For this review, take the finished solid that the model builds, in its own axes (mm). A direction names the side the tool comes from. Give positions to 0.01 mm unless a question says otherwise; leave off trailing zeros. Write each loop counter-clockwise with the first axis right and the second up, starting at its lowest first coordinate (ties: lowest second). Pieces come first, ordered by that corner, then holes.
1) We need section B-B on z = -22. Give the boundary of the cut face in (x, y), and give its area (3 significant figures).
2) We need section A-A on y = 0.7. Give the boundary of the cut face in (x, z), and give its area (3 significant figures).
3) Wall thickness on line 1 along Z through (x, y) = (4, 0.5); line 2 along X through (y, z) = (0.5, -3); line 3 along Z through (x, y) = (5.25, 0.7): over which ranges is each line inside the solid? List them lowest first.
4) For P1, Ø0.5, axis at x = 18, y = 0.5, coming from the +Z side; P2, Ø0.5, axis at y = 0.5, z = -1.5, coming from the +X side, all flat-tipped, find the tip position at first contact; note any pin that passes through.
5) Draft analysis for pull direction X (two halves, no side actions). For faces 3 (the face through (18.5, 0.5, -20.3)), 4 (the face through (2.25, 0.49, -3.08)), 5 (the face through (17.9, 0.5, -2.2)), state which applies: pulls with the +X half, pulls with the -X half, needs draft (parallel to the pull), parting line crosses it, or undercut.
6) We need section C-C on x = 4. Give the boundary of the cut face in (y, z), and give its area (3 significant figures).
7) Machinability: for faces 1 (the face through (17.3, 0.5, -1.1)), 2 (the face through (0.285, 0.507, -39.699)), which of the approach directions +Z, -Z, +X, -X, +Y, -Y give a long, thin tool a straight path to every point of the face, cutting with its end or side? Answer none if there is none.
from build123d import *

# Parameters (mm, degrees)
CROQUIS1_W              = 18.5
CROQUIS1_H              = 40
CROQUIS1_R              = 1.75
SALIENTE_EXTRUIR1_DEPTH = 1
CROQUIS2_W              = 1.2
CROQUIS2_H              = 2.2
CORTAR_EXTRUIR1_DEPTH   = 1
REDONDEO1_R             = 1


with BuildPart() as part:
    # Croquis1 → Saliente-Extruir1 (new body)
    with BuildSketch(Plane(origin=(0, 0, 0), x_dir=(1, 0, 0), z_dir=(0, 1, 0))):
        with Locations((9.25, 20)):
            Rectangle(CROQUIS1_W, CROQUIS1_H)
        with Locations((4, 3)):
            Circle(CROQUIS1_R, mode=Mode.SUBTRACT)
        with Locations((4, 22)):
            Circle(CROQUIS1_R, mode=Mode.SUBTRACT)
    extrude(amount=SALIENTE_EXTRUIR1_DEPTH)

    # Croquis2 → Cortar-Extruir1 (cut)
    with BuildSketch(Plane(origin=(0, 1, 0), x_dir=(1, 0, 0), z_dir=(0, 1, 0))):
        with Locations((17.9, 1.1)):
            Rectangle(CROQUIS2_W, CROQUIS2_H)
    extrude(amount=-CORTAR_EXTRUIR1_DEPTH, mode=Mode.SUBTRACT)

    # Redondeo1
    redondeo1_edges = [part.edges().sort_by_distance(p)[0] for p in [
        (0, 0.5, -40),
        (18.5, 0.5, -40),
    ]]
    fillet(redondeo1_edges, radius=REDONDEO1_R)


solid = part.part
Results list:
1. outline: (0, 0) - (2.25, 0) - (2.25, 1) - (0, 1) - close; (5.75, 0) - (18.5, 0) - (18.5, 1) - (5.75, 1) - close
1. area: 15.0 mm2
2. outline: (0, -39) arc R1 ccw to (1, -40) - (17.5, -40) arc R1 ccw to (18.5, -39) - (18.5, -2.2) - (17.3, -2.2) - (17.3, 0) - (0, 0) - close; hole circle Ø3.5 at (4, -22); hole circle Ø3.5 at (4, -3)
2. area: 718 mm2
3. line 1: z = -40 to -23.75, -20.25 to -4.75, -1.25 to 0
3. line 2: x = 0 to 2.25, 5.75 to 18.5
3. line 3: z = -40 to -23.22, -20.78 to -4.22, -1.78 to 0
4. P1: stops at z = -2.2
4. P2: stops at x = 17.3
5. face 3: pulls with the +X half
5. face 4: undercut
5. face 5: needs draft
6. outline: (0, -40) - (1, -40) - (1, -23.75) - (0, -23.75) - close; (0, -20.25) - (1, -20.25) - (1, -4.75) - (0, -4.75) - close; (0, -1.25) - (1, -1.25) - (1, 0) - (0, 0) - close
6. area: 33.0 mm2
7. face 1: +Z, +X, +Y, -Y
7. face 2: -Z, -X, +Y, -Y
